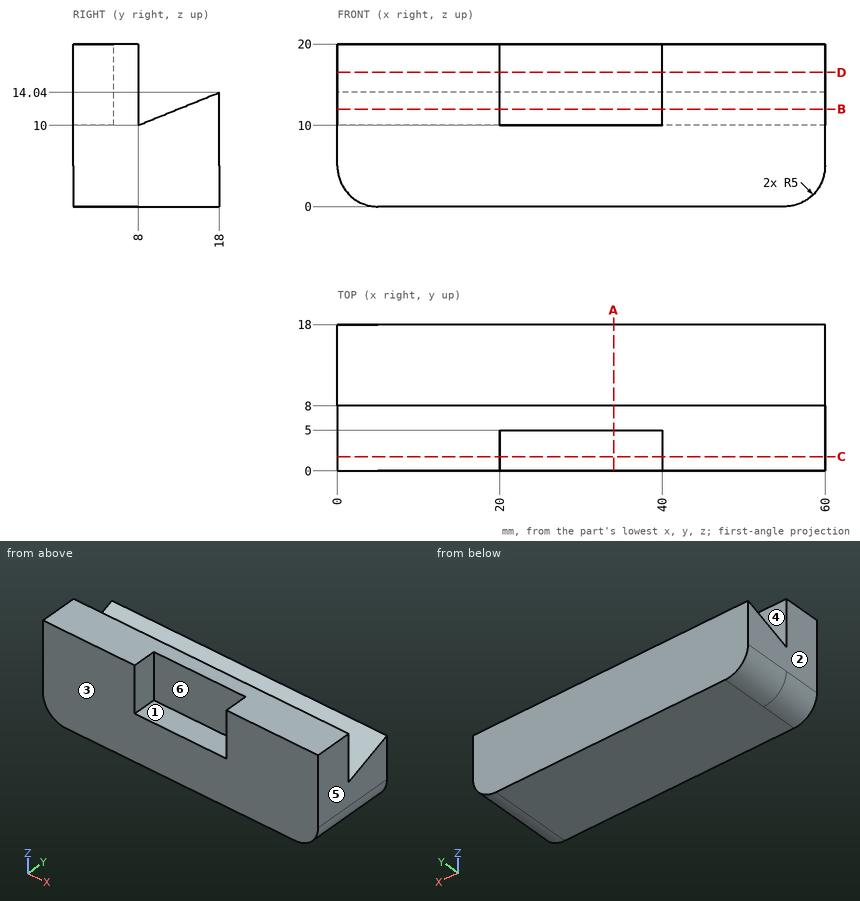
Geometry check sheet. Reference: drawing and pictorial views, mm from the part's lowest x, y, z. A direction names the side the tool comes from. Give positions to 0.01 mm unless a question says otherwise; leave off trailing zeros. Loops run counter-clockwise (first coordinate to the right, second up) from the corner with the lowest first, then second, coordinate; pieces in that order, holes last. Notation, with made-up numbers: (44.5, -8) -> (50.5, -8) arc R23 cw to (50.5, 31) -> close; hole circle Ø4 at (9, 39). An arc over 180 degrees is marked (long way). Answer in a Markdown table with one row per item. Add a question column.
1) Draft check along X on the marked faces 1, 2 and 3. Enter one of: pulls with the +X half, pulls with the -X half, needs draft (parallel to the pull), parting line crosses it, or undercut.
2) Set-up check for the marked faces 4, 5 and 6: record each of +Z, -Z, +X, -X, +Y, -Y from which the full face is reachable in a straight line by a thin tool's end or side.
3) Material ranges on probe 1 along X at (y, z) = (4.5, 17.5); probe 2 along Y at (x, z) = (31, 16); probe 3 along Z at (x, y) = (38, 4.25), recorded low to high. Write a range as from..to.
4) Cross-section at C-C on y = 1.75. Record the boundary of the cut face in (x, z), and give its area (3 significant figures).
5) Gauge pin test, flat ends, axial feed: P1, Ø6, axis at x = 53, z = 17, coming from the +Y side; P2, Ø1.5, axis at x = 30, y = 10.5, coming from the +Z side; P3, Ø8, axis at x = 27, z = 15, coming from the -Y side; P4, Ø2.5, axis at x = 30, y = 2.5, coming from the +Z side. Record the tip position at first contact, or that the pin passes through.
6) Cross-section at A-A on x = 34. Record the boundary of the cut face in (y, z), and give its area (3 significant figures).
7) Cross-section at D-D on z = 16.5. Record the boundary of the cut face in (x, y).
8) Cross-section at B-B on z = 12. Record the boundary of the cut face in (x, y).
Outcome:
| question | item | result |
|---|---|---|
| 1 | face 1 | undercut |
| 1 | face 2 | pulls with the -X half |
| 1 | face 3 | needs draft |
| 2 | face 4 | +Z, +X, -X |
| 2 | face 5 | +Z, -Z, +X, +Y, -Y |
| 2 | face 6 | +Z, -Y |
| 3 | probe 1 | x = 0..20, 40..60 |
| 3 | probe 2 | y = 5..8 |
| 3 | probe 3 | z = 0..10 |
| 4 | outline | (0, 5) arc R5 ccw to (5, 0) -> (55, 0) arc R5 ccw to (60, 5) -> (60, 20) -> (40, 20) -> (40, 10) -> (20, 10) -> (20, 20) -> (0, 20) -> close |
| 4 | area | 989 mm^2 |
| 5 | P1 | stops at y = 18 |
| 5 | P2 | stops at z = 11.31 |
| 5 | P3 | stops at y = 5 |
| 5 | P4 | stops at z = 10 |
| 6 | outline | (0, 0) -> (18, 0) -> (18, 14.04) -> (8, 10) -> (8, 20) -> (5, 20) -> (5, 10) -> (0, 10) -> close |
| 6 | area | 230 mm^2 |
| 7 | outline | (0, 0) -> (20, 0) -> (20, 5) -> (40, 5) -> (40, 0) -> (60, 0) -> (60, 8) -> (0, 8) -> close |
| 8 | outline | (0, 0) -> (20, 0) -> (20, 5) -> (40, 5) -> (40, 0) -> (60, 0) -> (60, 8) -> (0, 8) -> close; (0, 12.95) -> (60, 12.95) -> (60, 18) -> (0, 18) -> close |
